Could you check a few things on this model? Use its own coordinates, in mm. Face numbers are marked on the shaded views. Coordinates: 2 decimals unless noted, no trailing zeros. Write each loop counter-clockwise with the first axis right and the second up, starting at its lowest first coordinate (ties: lowest second). Pieces come first, ordered by that corner, then holes.
```python
from build123d import *

# Parameters (mm, degrees)
ESQUISSE1_W             = 10
ESQUISSE1_H             = 14
BOSS_EXTRU_1_DEPTH      = 1
ESQUISSE2_W             = 10
ESQUISSE2_H             = 14
ESQUISSE2_W_2           = 8
ESQUISSE2_H_2           = 12
BOSS_EXTRU_2_DEPTH      = 20
ESQUISSE3_R             = 1
ENL_V_MAT_EXTRU_1_DEPTH = 44.02494538
ESQUISSE4_R             = 1
ENL_V_MAT_EXTRU_2_DEPTH = 53.662523212


with BuildPart() as part:
    # Esquisse1 → Boss.-Extru.1 (new body)
    with BuildSketch(Plane.XY):
        with Locations((-41.220572811, -29.195937962)):
            Rectangle(ESQUISSE1_W, ESQUISSE1_H)
    extrude(amount=BOSS_EXTRU_1_DEPTH)

    # Esquisse2 → Boss.-Extru.2 (add)
    with BuildSketch(Plane.XY.offset(1)):
        with Locations((-41.220572811, -29.195937962)):
            Rectangle(ESQUISSE2_W, ESQUISSE2_H)
        with Locations((-41.220572811, -29.195937962)):
            Rectangle(ESQUISSE2_W_2, ESQUISSE2_H_2, mode=Mode.SUBTRACT)
    extrude(amount=BOSS_EXTRU_2_DEPTH)

    # Esquisse3 → Enlèv. mat.-Extru.1 (cut, through all)
    with BuildSketch(Plane.ZY.offset(46.220572811)):
        with Locations(Location((3.252145139, -27.044676275, 0), (0, 0, 270))):
            Circle(ESQUISSE3_R)
        with Locations(Location((10.430913125, -27.044676275, 0), (0, 0, 270))):
            Circle(ESQUISSE3_R)
        with Locations(Location((6.720877569, -30.948290196, 0), (0, 0, 270))):
            Circle(ESQUISSE3_R)
        with Locations(Location((10.430913125, -30.948290196, 0), (0, 0, 270))):
            Circle(ESQUISSE3_R)
        with Locations(Location((14.321926026, -30.948290196, 0), (0, 0, 270))):
            Circle(ESQUISSE3_R)
        with Locations(Location((14.321926026, -27.044676275, 0), (0, 0, 270))):
            Circle(ESQUISSE3_R)
        with Locations(Location((6.720877569, -27.044676275, 0), (0, 0, 270))):
            Circle(ESQUISSE3_R)
        with Locations(Location((3.252145139, -30.948290196, 0), (0, 0, 270))):
            Circle(ESQUISSE3_R)
    extrude(amount=-ENL_V_MAT_EXTRU_1_DEPTH, mode=Mode.SUBTRACT)

    # Esquisse4 → Enlèv. mat.-Extru.2 (cut, through all)
    with BuildSketch(Plane(origin=(0, -22.195937962, 0), x_dir=(1, 0, 0), z_dir=(0, 1, 0))):
        with Locations(Location((-41.257446794, -3.10676642, 0), (0, 0, 270))):
            Circle(ESQUISSE4_R)
        with Locations(Location((-41.257446794, -6.425424885, 0), (0, 0, 270))):
            Circle(ESQUISSE4_R)
        with Locations(Location((-41.257446794, -9.780957333, 0), (0, 0, 270))):
            Circle(ESQUISSE4_R)
        with Locations(Location((-41.257446794, -13.320859695, 0), (0, 0, 270))):
            Circle(ESQUISSE4_R)
    extrude(amount=-ENL_V_MAT_EXTRU_2_DEPTH, mode=Mode.SUBTRACT)


solid = part.part
```
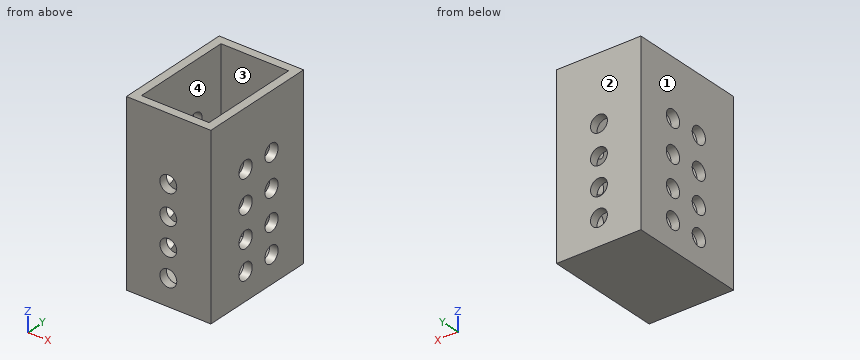
Item 1: I want a section at C-C, the plane x = -43. List the corners of the cut face in (y, z) for me.
Item 2: I want a section at D-D, the plane z = 10. Count the separate pieces of the cut face and the enclosed holes in it, then the cut area to 3 significant figures.
Item 3: I want a section at B-B, the plane y = -34.75. List the corners of the cut face in (x, z) for me, then the cut area to 3 significant figures.
Item 4: If I drill on line 1 along Y through (x, z) = (-42, 18.25); line 2 along X through (y, z) = (-34.25, 16.75); line 3 along Z through (x, y) = (-37.5, -34), over which ranges is the centre line in solid material (lowest first)?
Item 5: I want a section at A-A, the plane z = 19.75. List the corners of the cut face in (x, y) for me.
Item 6: Will this pin go through, and if not, where does the flat tip stop? pin 1 Ø1.8 at (x, z) = (-41.26, 13.32) entering from -Y.
Item 7: If we mould it in two halves opening along X, with no side actions, what happens to the marked faces 1, 2, 3 and 4? For each: released by +X, released by -X, zero draft, split by the parting line, or undercut.
Taken from the geometry:
1. outline: (-36.2, 0) - (-22.2, 0) - (-22.2, 21) - (-23.2, 21) - (-23.2, 1) - (-35.2, 1) - (-35.2, 21) - (-36.2, 21) - close
2. separate pieces: 6
2. enclosed holes: 0
2. area: 32.9 mm2
3. outline: (-46.22, 0) - (-36.22, 0) - (-36.22, 21) - (-37.22, 21) - (-37.22, 1) - (-45.22, 1) - (-45.22, 21) - (-46.22, 21) - close
3. area: 50.0 mm2
4. line 1: y = -36.2 to -35.2, -23.2 to -22.2
4. line 2: x = -46.22 to -45.22, -37.22 to -36.22
4. line 3: z = 0 to 1
5. outline: (-46.22, -36.2) - (-36.22, -36.2) - (-36.22, -22.2) - (-46.22, -22.2) - close; hole (-45.22, -35.2) - (-37.22, -35.2) - (-37.22, -23.2) - (-45.22, -23.2) - close
6. pin 1: passes through
7. face 1: released by -X
7. face 2: zero draft
7. face 3: undercut
7. face 4: undercut
